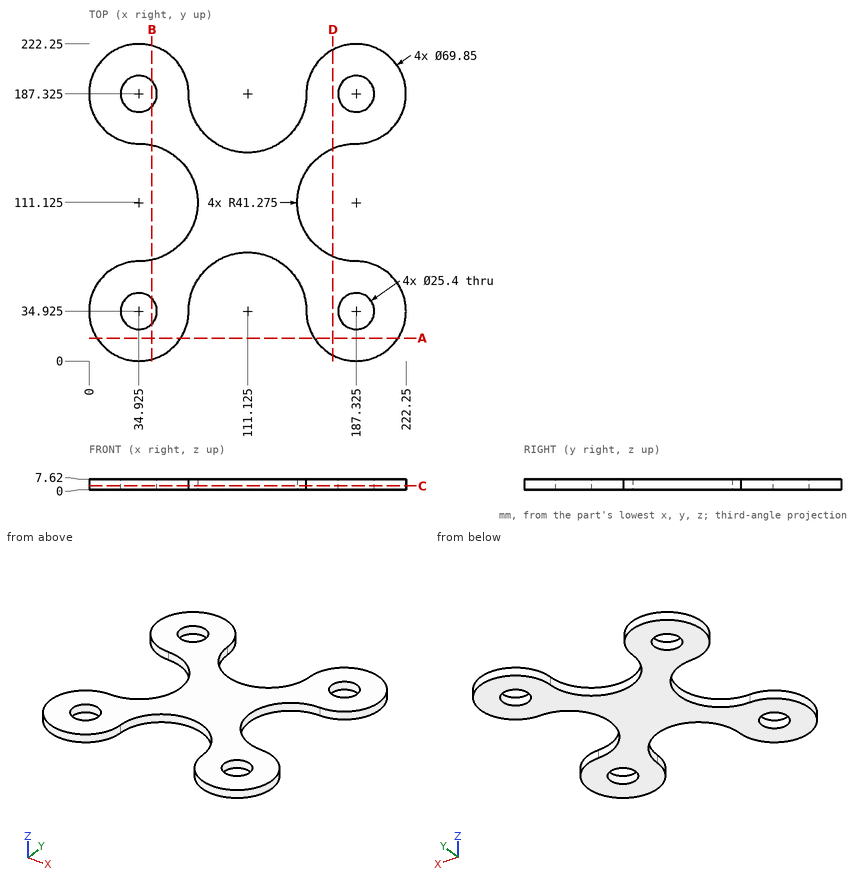
Job drawing, mm, ordinate dimensions from the low corner. One solid piece. Coordinates: 2 decimals unless noted, no trailing zeros. Write each loop counter-clockwise with the first axis right and the second up, starting at its lowest first coordinate (ties: lowest second). Pieces come first, ordered by that corner, then holes. Notation, with made-up numbers: M -24,10 L -11,10 A34 cw -11,48 Z; hole C 64.5,38.5 d10. An arc over 180 degrees is marked long. Answer as a JSON object with one key per item and string values. Group by question number.
1) Saw through at B-B (x = 44). Write the cut outline in (y, z), plus the area to 3 significant figures.
2) Saw through at A-A (y = 16). Write the cut outline in (x, z).
3) Saw through at D-D (x = 171). Write the cut outline in (y, z).
4) Saw through at C-C (z = 2.75). Write the cut outline in (x, y) (3 decimals), plus the area to 3 significant figures.
5) Wall check: line 1 (X direction, y = 187, z = 2.25); line 2 (Y direction, x = 195.5, z = 6.5); line 3 (Y direction, x = 167, z = 1.5). Give the ranges that are in metal, low to high. Write a range as from..to.
6) Pin check, flat tips, straight feed: pin 1 Ø3 at (x, z) = (122, 4) entering from +Y; pin 2 Ø1 at (x, y) = (143.5, 135) entering from -Z; pin 3 Ø1.5 at (y, z) = (75, 4.5) entering from -X; pin 4 Ø3 at (y, z) = (103.5, 3.5) entering from -X. Stop position of each tip, or through.
Values follow:
{
 "1": {"outline": "M 1.2,0 L 26.04,0 L 26.04,7.62 L 1.2,7.62 Z; M 43.81,0 L 70.86,0 L 70.86,7.62 L 43.81,7.62 Z; M 151.39,0 L 178.44,0 L 178.44,7.62 L 151.39,7.62 Z; M 196.21,0 L 221.05,0 L 221.05,7.62 L 196.21,7.62 Z", "area": "791 mm2"},
 "2": {"outline": "M 5.57,0 L 64.28,0 L 64.28,7.62 L 5.57,7.62 Z; M 157.97,0 L 216.68,0 L 216.68,7.62 L 157.97,7.62 Z"},
 "3": {"outline": "M 4.05,0 L 73.22,0 L 73.22,7.62 L 4.05,7.62 Z; M 149.03,0 L 218.2,0 L 218.2,7.62 L 149.03,7.62 Z"},
 "4": {"outline": "M 34.925,69.85 A34.925 ccw long 69.85,34.925 A41.275 cw 152.4,34.925 A34.925 ccw long 187.325,69.85 A41.275 cw 187.325,152.4 A34.925 ccw long 152.4,187.325 A41.275 cw 69.85,187.325 A34.925 ccw long 34.925,152.4 A41.275 cw Z; hole C 34.925,34.925 d25.4; hole C 34.925,187.325 d25.4; hole C 187.325,34.925 d25.4; hole C 187.325,187.325 d25.4", "area": "22,000 mm2"},
 "5": {"line 1": "x = 0..22.23, 47.62..69.85, 152.4..174.63, 200.02..222.25", "line 2": "y = 0.97..25.21, 44.64..68.88, 153.37..177.61, 197.04..221.28", "line 3": "y = 6.52..75.2, 147.05..215.73"},
 "6": {"pin 1": "stops at y = 147.95", "pin 2": "stops at z = 0", "pin 3": "stops at x = 53.47", "pin 4": "stops at x = 75.18"}
}
